The model under review builds one solid part; all positions refer to its coordinate system, in mm. Give positions to 0.01 mm unless a question says otherwise; leave off trailing zeros. Write each loop counter-clockwise with the first axis right and the second up, starting at its lowest first coordinate (ties: lowest second). Pieces come first, ordered by that corner, then holes.
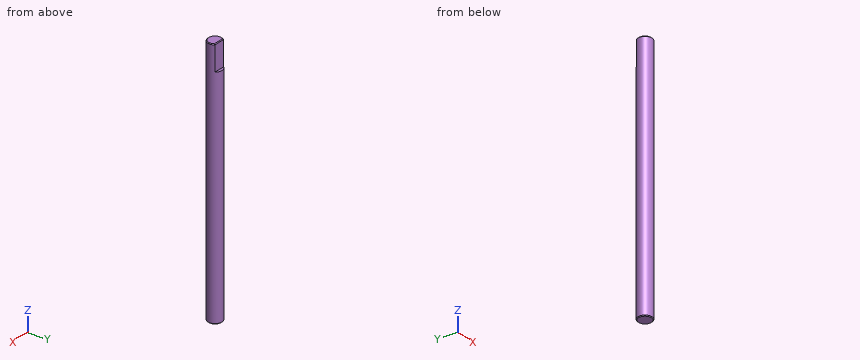
from build123d import *

# Parameters (mm, degrees)
SKETCH1_R           = 2.5
BOSS_EXTRUDE1_DEPTH = 90
CUT_EXTRUDE1_DEPTH  = 9
CHAMFER1_SIZE       = 0.25


with BuildPart() as part:
    # Sketch1 → Boss-Extrude1 (new body)
    with BuildSketch(Plane.XY):
        with Locations(Location((0, 0, 0), (0, 0, 180))):
            Circle(SKETCH1_R)
    extrude(amount=BOSS_EXTRUDE1_DEPTH)

    # Sketch2 → Cut-Extrude1 (cut)
    with BuildSketch(Plane.XY.offset(90)):
        with BuildLine():
            Line((-2.454110015, 1.5), (2.151792115, 1.5))
            ThreePointArc((2.151792115, 1.5), (-0.15115895, 4.391411645), (-2.454110015, 1.5))
        make_face()
    extrude(amount=-CUT_EXTRUDE1_DEPTH, mode=Mode.SUBTRACT)

    # Chamfer1
    chamfer1_edges = [part.edges().sort_by_distance(p)[0] for p in [
        (2.5, 0, 0),
        (0.790569415, -2.371708245, 90),
        (0, 1.5, 90),
    ]]
    chamfer(chamfer1_edges, length=CHAMFER1_SIZE)


solid = part.part
1) Consider section B-B, the plane z = 35. Give the boundary of the cut face in (x, y), then the cut area to 3 significant figures.
2) Insertion check: pin 1 (1.1 mm diameter, centred on x = -0.5, y = 2, fed in from +Z). The pin has a flat end and moves straight along its axis. Give the tip position at first contact, or say it passes through.
3) Consider section A-A, the plane x = 0. Give the boundary of the cut face in (y, z), then the cut area to 3 significant figures.
4) To check wall thickness, follow probe 1 along X at (y, z) = (-0.25, 67.5); probe 2 along Y at (x, z) = (1.05, 78); probe 3 along Y at (x, z) = (2.05, 83). State the ranges of each line that lie inside material, in increasing order.
Answer block:
1. outline: circle Ø5 at (0, 0)
1. area: 19.6 mm2
2. pin 1: stops at z = 89.8
3. outline: (-2.5, 0.25) - (-2.25, 0) - (2.25, 0) - (2.5, 0.25) - (2.5, 81) - (1.5, 81) - (1.5, 89.75) - (1.25, 90) - (-2.25, 90) - (-2.5, 89.75) - close
3. area: 441 mm2
4. probe 1: x = -2.49 to 2.49
4. probe 2: y = -2.27 to 2.27
4. probe 3: y = -1.43 to 1.43
